Model file for the job. Use its own axes, mm. A direction names the side the tool comes from. Coordinates: 2 decimals unless noted, no trailing zeros. Write each loop counter-clockwise with the first axis right and the second up, starting at its lowest first coordinate (ties: lowest second). Pieces come first, ordered by that corner, then holes. Notation, with made-up numbers: (-21, -23.75) - (-15, -23.75) arc R34 cw to (-15, 12.25) - close; hole circle Ø5 at (-38, 29.25). An arc over 180 degrees is marked (long way). Put each result on its own line as item: value. Start each with the question number.
1. Pull direction X, two halves, no side cores. Call faces 1 (the face through (0, 20, -13)), 2 (the face through (12, 20, 0)), 3 (the face through (11.69, 33.45, -0.99)), 4 (the face through (25, 20, -1)): released by +X, released by -X, zero draft, split by the parting line, or undercut.
2. Which spindle directions (+Z, -Z, +X, -X, +Y, -Y) get a long thin tool onto all of the face, cutting with end or side? Do faces 5 (the face through (2, 20, -13)), 6 (the face through (1, 0, -7)). Say none if no direction does.
3. Drill centre lines: L1, parallel to Y at x = 1.1, z = -10; L2, parallel to Y at x = 12.5, z = -0.8; L3, parallel to Z at x = 1.5, y = 5. Where is each one in solid material? Low to high. Write a range as from..to.
4. Saw through at B-B, the plane y = 35. Write the cut outline in (x, z), plus the area to 3 significant figures.
5. Saw through at A-A, the plane z = -10. Write the cut outline in (x, y).
6. Drop flat-ended pins along their axis: P1, Ø12, axis at y = 34, z = -19.5, coming from the +X side; P2, Ø10, axis at x = 15.5, z = -9.5, coming from the +Y side. Give the stop position or say it passes through.
7. Saw through at C-C, the plane x = 13. Write the cut outline in (y, z), plus the area to 3 significant figures.
8. Saw through at D-D, the plane y = 30. Write the cut outline in (x, z).
```python
from build123d import *

# Parameters (mm, degrees)
BOSS_EXTRUDE1_DEPTH = 40
SKETCH2_R           = 1.75
CUT_EXTRUDE1_DEPTH  = 50
SKETCH3_R           = 1.75
CUT_EXTRUDE2_DEPTH  = 50


with BuildPart() as part:
    # Sketch1 → Boss-Extrude1 (new body)
    with BuildSketch(Plane(origin=(0, 0, 0), x_dir=(1, 0, 0), z_dir=(0, 1, 0))):
        Polygon((0, 0), (25, 0), (25, 2), (2, 2), (2, 25), (0, 25), align=None)
    extrude(amount=BOSS_EXTRUDE1_DEPTH)

    # Sketch2 → Cut-Extrude1 (cut)
    with BuildSketch(Plane(origin=(0, 0, 0), x_dir=(0, 0, -1), z_dir=(1, 0, 0))):
        with Locations((10, 5)):
            Circle(SKETCH2_R)
    extrude(amount=CUT_EXTRUDE1_DEPTH, mode=Mode.SUBTRACT)

    # Sketch3 → Cut-Extrude2 (cut)
    with BuildSketch(Plane(origin=(0, 0, 0), x_dir=(-1, 0, 0), z_dir=(0, 0, -1))):
        with Locations((-12.5, 35)):
            Circle(SKETCH3_R)
    extrude(amount=CUT_EXTRUDE2_DEPTH, mode=Mode.SUBTRACT)


solid = part.part
```
Final values:
1. face 1: released by -X
1. face 2: zero draft
1. face 3: undercut
1. face 4: released by +X
2. face 5: -Z, +X, +Y, -Y
2. face 6: +Z, -Z, +X, -X, -Y
3. L1: y = 0..3.25, 6.75..40
3. L2: y = 0..33.25, 36.75..40
3. L3: z = -25..-11.75, -8.25..0
4. outline: (0, -25) - (2, -25) - (2, -2) - (10.75, -2) - (10.75, 0) - (0, 0) - close; (14.25, -2) - (25, -2) - (25, 0) - (14.25, 0) - close
4. area: 89.0 mm²
5. outline: (0, 0) - (2, 0) - (2, 3.25) - (0, 3.25) - close; (0, 6.75) - (2, 6.75) - (2, 40) - (0, 40) - close
6. P1: stops at x = 2
6. P2: passes through
7. outline: (0, -2) - (33.32, -2) - (33.32, 0) - (0, 0) - close; (36.68, -2) - (40, -2) - (40, 0) - (36.68, 0) - close
7. area: 73.3 mm²
8. outline: (0, -25) - (2, -25) - (2, -2) - (25, -2) - (25, 0) - (0, 0) - close
